Build history of the part. All positions in model axes, mm. A direction names the side the tool comes from. Give positions to 0.01 mm unless a question says otherwise; leave off trailing zeros. Write each loop counter-clockwise with the first axis right and the second up, starting at its lowest first coordinate (ties: lowest second). Pieces come first, ordered by that corner, then holes. Notation, with made-up numbers: (9.5, 26.5) -> (67.5, 26.5) arc R23 cw to (67.5, 41.5) -> close; hole circle Ø4 at (4, 4.5). An arc over 180 degrees is marked (long way). One line per question, with ' | ' between items. Start each with the question number.
(1) Drill centre lines: probe 1 along Z at (x, y) = (0, 2.1); probe 2 along Z at (x, y) = (9.25, 3.5); probe 3 along X at (y, z) = (2.1, 152). Where is each one in solid material? Low to high. Write a range as from..to.
(2) Band-saw the part on B-B, the plane z = 21.5. Give the cut face in (x, y), and give its area (3 significant figures).
(3) Tool access for faces 1 (the flat face through (-3.045, 4.491, 153.726)), 2 (the flat face through (0, 5.6, 75)), 3 (the flat face through (9.425, 5, 153)): list every direction of +Z, -Z, +X, -X, +Y, -Y with a clear straight run to the whole face (end or side of a thin tool).
(4) Pull direction Z, two halves, no side cores. Call faces 4 (the flat face through (-6.05, 1.19, 144.97)), 5 (the flat face through (0, 5, 20)), 6 (the cylindrical face through (0.1, 5.31, 144.97)), 7 (the flat face through (9.425, 5, 48)): released by +Z, released by -Z, zero draft, split by the parting line, or undercut.
(5) Pin check, flat tips, straight feed: P1, Ø3, axis at y = 5, z = 42.5, coming from the +X side; P2, Ø0.8, axis at y = 5, z = 47.5, coming from the -X side; P3, Ø3, axis at y = 4.5, z = 101.5, coming from the +X side. Stop position of each tip, or through.
(6) Band-saw the part on A-A, the plane x = 0. Give the cut face in (y, z).
from build123d import *

# Parameters (mm, degrees)
EXTRUDE_1_DEPTH                  = 160
SKETCH_4_W                       = 18.849551718
SKETCH_4_H                       = 140
EXTRUDE_2_DEPTH                  = 2.78
CUT_EXTRUDE_2_DEPTH              = 161.420208827
CUT_EXTRUDE_2_DEPTH_BACK         = 161.420208827
SKETCH_5_R                       = 1.95
CUT_EXTRUDE_3_DEPTH              = 3
CHAMFER_1_SIZE                   = 1
SKETCH_8_W                       = 4
SKETCH_8_H                       = 1
CUT_EXTRUDE_4_DEPTH              = 161.481311685
CUT_EXTRUDE_5_DEPTH              = 4
FILLET_1_R                       = 1
PATTERN_LINEAR_1_COUNT           = 2
PATTERN_LINEAR_1_PITCH           = 68
PATTERN_LINEAR_1_COPY_1_SKETCH_W = 4
PATTERN_LINEAR_1_COPY_1_SKETCH_H = 1
PATTERN_LINEAR_1_COPY_1_DEPTH    = 161.481311685
FILLET_1_OF_PATTERN_LINEAR_1_R   = 1


with BuildPart() as part:
    # 스케치1 → 보스-돌출1 (new body)
    with BuildSketch(Plane.XY):
        with BuildLine():
            Line((-9.424775859, 3.19), (9.424775859, 3.19))
            ThreePointArc((9.424775859, 3.19), (9.936964373, 0.509155237), (9.701463807, -2.21))
            Line((9.701463807, -2.21), (5.65, -2.21))
            Line((5.65, -2.21), (4.15, -0.71))
            Line((4.15, -0.71), (-4.15, -0.71))
            Line((-4.15, -0.71), (-5.65, -2.21))
            Line((-5.65, -2.21), (-9.701463807, -2.21))
            ThreePointArc((-9.701463807, -2.21), (-9.936964373, 0.509155237), (-9.424775859, 3.19))
        make_face()
    extrude(amount=EXTRUDE_1_DEPTH)

    # 스케치4 → 보스-돌출2 (add)
    with BuildSketch(Plane(origin=(0, 3.19, 0), x_dir=(1, 0, 0), z_dir=(0, 1, 0))):
        with Locations((0, -90)):
            Rectangle(SKETCH_4_W, SKETCH_4_H)
    extrude(amount=EXTRUDE_2_DEPTH)

    # 스케치5 → 컷-돌출2 (cut, two sides: drawn at the far end of the back side and taken through both)
    with BuildSketch(Plane(origin=(0, 0, 0), x_dir=(1, 0, 0), z_dir=(0, 1, 0)).offset(-CUT_EXTRUDE_2_DEPTH_BACK)):
        with Locations(Location((0, -152, 0), (0, 0, 180))):
            Circle(SKETCH_5_R)
    extrude(amount=CUT_EXTRUDE_2_DEPTH + CUT_EXTRUDE_2_DEPTH_BACK, mode=Mode.SUBTRACT)

    # 스케치6 → 컷-돌출3 (cut)
    with BuildSketch(Plane(origin=(0, 5.97, 0), x_dir=(1, 0, 0), z_dir=(0, 1, 0))):
        Polygon((4.041451884, -152), (2.020725942, -148.5), (-2.020725942, -148.5), (-4.041451884, -152), (-2.020725942, -155.5), (2.020725942, -155.5), align=None)
    extrude(amount=-CUT_EXTRUDE_3_DEPTH, mode=Mode.SUBTRACT)

    # 모따기1
    chamfer_1_edges = [part.edges().sort_by_distance(p)[0] for p in [
        (0, -0.71, 160),
        (-4.9, -1.46, 160),
        (-7.675731904, -2.21, 160),
        (-9.936964373, 0.509155237, 160),
        (-9.424775859, 4.58, 160),
        (0, 5.97, 160),
        (9.424775859, 4.58, 160),
        (9.936964373, 0.509155237, 160),
        (7.675731904, -2.21, 160),
        (4.9, -1.46, 160),
    ]]
    chamfer(chamfer_1_edges, length=CHAMFER_1_SIZE)

    # 스케치8 → 컷-돌출4 (cut, through all)
    with BuildSketch(Plane(origin=(1.72, 1.72, 0), x_dir=(0, 0, 1), z_dir=(-0.7071067811865488, -0.7071067811865464, 0))):
        with Locations((77, -3.936538957)):
            Rectangle(SKETCH_8_W, SKETCH_8_H)
    cut_extrude_4 = extrude(amount=-CUT_EXTRUDE_4_DEPTH, mode=Mode.SUBTRACT)

    # 대칭 복사1: 컷-돌출4 across plane
    add(cut_extrude_4.mirror(Plane(origin=(0, 0, 0), x_dir=(0, 0, 1), z_dir=(1, 0, 0))), mode=Mode.SUBTRACT)

    # 스케치9 → 컷-돌출5 (cut)
    with BuildSketch(Plane.XY.offset(75)):
        with BuildLine():
            Line((-9.424775859, 4.564775859), (-13.291839, 9.783941573))
            Line((-13.291839, 9.783941573), (12.328532893, 9.783941573))
            Line((12.328532893, 9.783941573), (9.424775859, 4.564775859))
            ThreePointArc((9.424775859, 4.564775859), (0, 5.311625169), (-9.424775859, 4.564775859))
        make_face()
    cut_extrude_5 = extrude(amount=CUT_EXTRUDE_5_DEPTH, mode=Mode.SUBTRACT)

    # 필렛1
    # the kernel refuses this fillet: 1 mm, written as the material it takes off along each edge
    with BuildSketch(Plane(origin=(9.424775859, 4.564775859, 79), x_dir=(-0.7071067811865487, -0.7071067811865465, 0), z_dir=(0, 0, -1))) as fillet_1_piece_1:
        with BuildLine():
            CenterArc((2.001337163, 1), FILLET_1_R, 142.129139592, 127.870860408)
            ThreePointArc((1.211940766, 1.613883807), (0.5991659, 0.812051708), (0, 0))
            Line((0, 0), (2.001337163, 0))
        make_face()
    extrude(amount=4, mode=Mode.SUBTRACT)
    with BuildSketch(Plane(origin=(-9.424775859, 4.564775859, 79), x_dir=(0.7071067811865489, -0.7071067811865462, 0), z_dir=(0, 0, -1))) as fillet_1_piece_2:
        with BuildLine():
            CenterArc((2.001337163, -1), FILLET_1_R, 90, 127.870860408)
            ThreePointArc((1.211940766, -1.613883807), (0.5991659, -0.812051708), (0, 0))
            Line((0, 0), (2.001337163, 0))
        make_face()
    extrude(amount=4, mode=Mode.SUBTRACT)

    # 선형 패턴1: 컷-돌출4, 컷-돌출5 ×2
    with Locations(*[(0, 0, i * PATTERN_LINEAR_1_PITCH) for i in range(1, PATTERN_LINEAR_1_COUNT)]):
        add(cut_extrude_4, mode=Mode.SUBTRACT)
        add(cut_extrude_5, mode=Mode.SUBTRACT)

    # 선형 패턴1 copy 1 sketch → 선형 패턴1 copy 1 (cut, through all)
    with BuildSketch(Plane(origin=(-1.72, 1.72, 68), x_dir=(0, 0, 1), z_dir=(0.7071067811865488, -0.7071067811865464, 0))):
        with Locations((77, 3.936538957)):
            Rectangle(PATTERN_LINEAR_1_COPY_1_SKETCH_W, PATTERN_LINEAR_1_COPY_1_SKETCH_H)
    extrude(amount=-PATTERN_LINEAR_1_COPY_1_DEPTH, mode=Mode.SUBTRACT)

    # 필렛1 of 선형 패턴1
    # the kernel refuses this fillet: 1 mm, written as the material it takes off along each edge
    with BuildSketch(Plane(origin=(9.424775859, 4.564775859, 147), x_dir=(-0.7071067811865485, -0.7071067811865467, 0), z_dir=(0, 0, -1)), Plane(origin=(-9.424775859, 4.564775859, 143), x_dir=(0.707106781186548, -0.7071067811865471, 0), z_dir=(0, 0, 1))) as fillet_1_of_pattern_linear_1_piece_1:
        with BuildLine():
            CenterArc((2.001337163, 1), FILLET_1_OF_PATTERN_LINEAR_1_R, 142.129139592, 127.870860408)
            ThreePointArc((1.211940766, 1.613883807), (0.5991659, 0.812051708), (0, 0))
            Line((0, 0), (2.001337163, 0))
        make_face()
    extrude(amount=4, mode=Mode.SUBTRACT)


solid = part.part
Results:
1) probe 1: z = 0..150.05, 153.95..160 | probe 2: z = 20..75, 79..143, 147..159.17 | probe 3: x = -9.73..-1.95, 1.95..9.73
2) outline: (-9.7, -2.21) -> (-5.65, -2.21) -> (-4.15, -0.71) -> (4.15, -0.71) -> (5.65, -2.21) -> (9.7, -2.21) arc R9.95 ccw to (9.42, 3.19) -> (9.42, 5.97) -> (-9.42, 5.97) -> (-9.42, 3.19) arc R9.95 ccw to start | area: 144 mm²
3) face 1: +Y | face 2: none | face 3: +Z, -Z, +X, +Y
4) face 4: undercut | face 5: released by -Z | face 6: undercut | face 7: zero draft
5) P1: stops at x = 9.42 | P2: stops at x = -9.42 | P3: stops at x = 9.49
6) outline: (-0.71, 0) -> (3.19, 0) -> (3.19, 20) -> (5.97, 20) -> (5.97, 75) -> (5.31, 75) -> (5.31, 79) -> (5.97, 79) -> (5.97, 143) -> (5.31, 143) -> (5.31, 147) -> (5.97, 147) -> (5.97, 148.5) -> (2.97, 148.5) -> (2.97, 150.05) -> (-0.71, 150.05) -> close; (-0.71, 153.95) -> (2.97, 153.95) -> (2.97, 155.5) -> (5.97, 155.5) -> (5.97, 159) -> (4.97, 160) -> (0.29, 160) -> (-0.71, 159) -> close
